Can you work these out from the drawing? Everything is in mm from the part's minimum corner. Give positions to 0.01 mm unless a question says otherwise; leave off trailing zeros. Write each loop counter-clockwise with the first axis right and the second up, starting at its lowest first coordinate (ties: lowest second). Pieces come first, ordered by that corner, then holes. Notation, with made-up numbers: (-24.75, 61) -> (12.25, 61) arc R24 ccw to (12.25, 92) -> close; hole circle Ø7 at (21.25, -25). An arc over 180 degrees is marked (long way). Use one line per item in the form item = value.
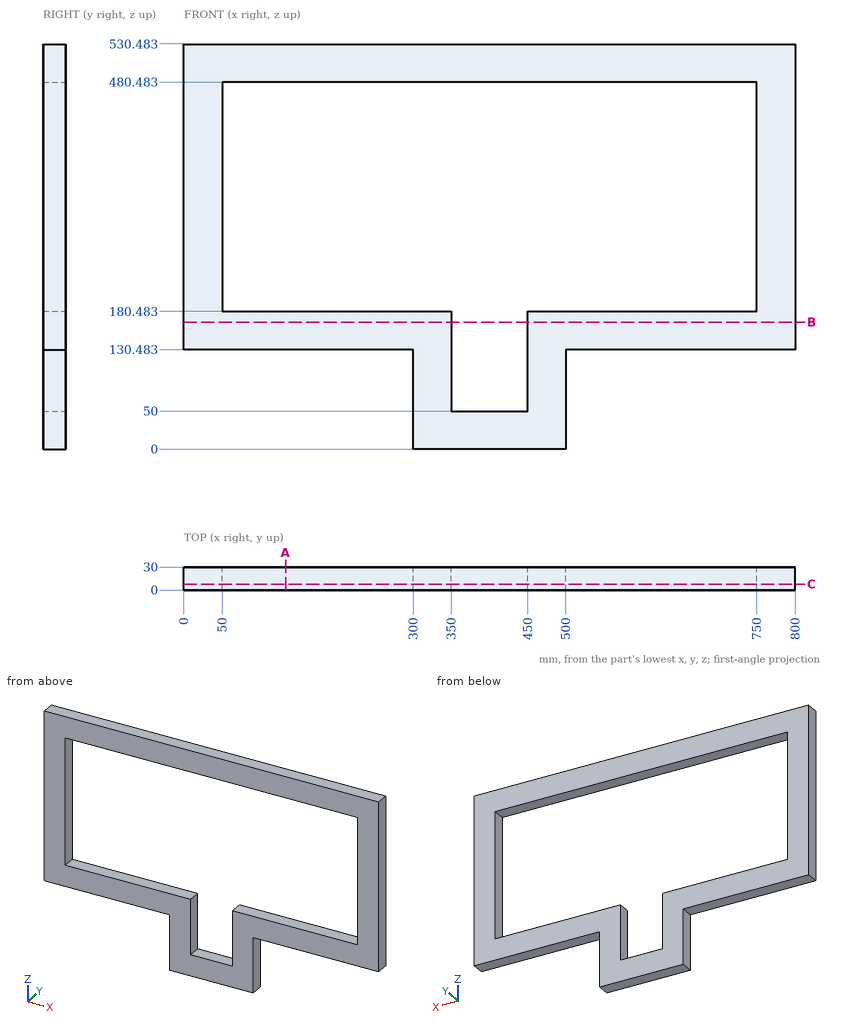
Q1. I want a section at B-B, the plane z = 166.5. Write out the boundary of the cut face in (x, y), and give its area (3 significant figures).
Result set:
outline = (0, 0) -> (350, 0) -> (350, 30) -> (0, 30) -> close; (450, 0) -> (800, 0) -> (800, 30) -> (450, 30) -> close
area = 21,000 mm2
Q2. Will these pins go through, and if not, where does the flat tip stop? pin 1 Ø8 at (x, z) = (561.5, 180.5) entering from -Y; pin 2 Ø9 at (y, z) = (13, 111) entering from +X; pin 3 Ø2 at (x, y) = (649.5, 14) entering from -Z; pin 4 Ø12 at (y, z) = (16.5, 99) entering from -X.
Result set:
pin_1 = 0
pin_2 = 500
pin_3 = 130.48
pin_4 = 300
Q3. If I drill on line 1 along Z through (x, y) = (283, 25.25); line 2 along X through (y, z) = (29, 458); line 3 along Z through (x, y) = (334, 17.5), over which ranges is the centre line in solid material (lowest first)? Write a range as from..to.
Result set:
line_1 = 130.48..180.48, 480.48..530.48
line_2 = 0..50, 750..800
line_3 = 0..180.48, 480.48..530.48
Q4. I want a section at A-A, the plane x = 133. Write out the boundary of the cut face in (y, z).
Result set:
outline = (0, 130.48) -> (30, 130.48) -> (30, 180.48) -> (0, 180.48) -> close; (0, 480.48) -> (30, 480.48) -> (30, 530.48) -> (0, 530.48) -> close
Q5. I want a section at C-C, the plane y = 8. Write out the boundary of the cut face in (x, z).
Result set:
outline = (0, 130.48) -> (300, 130.48) -> (300, 0) -> (500, 0) -> (500, 130.48) -> (800, 130.48) -> (800, 530.48) -> (0, 530.48) -> close; hole (50, 180.48) -> (350, 180.48) -> (350, 50) -> (450, 50) -> (450, 180.48) -> (750, 180.48) -> (750, 480.48) -> (50, 480.48) -> close
